Autodesk Fusion 360 part; units mm, degrees
sketch "Sketch1" plane through (0, 0, 0) normal (0, 0, 1) x (1, 0, 0)
  circle A0 centre (0, 0) radius 30
  dimension "d1" = 60
extrude "Extrude1" add sketch "Sketch1" along normal blind 5
sketch "Sketch2" plane through (0, 0, 5) normal (0, 0, 1) x (-1, 0, 0)
  circle A0 centre (0, 0) radius 30
  circle A1 centre (0, 0) radius 24.2
  dimension "d4" = 48.4
extrude "Extrude2" add sketch "Sketch2" along normal blind 25 contours A1
sketch "Sketch3" plane through (0, 0, 0) normal (0, 0, -1) x (1, 0, 0)
  circle A0 centre (0, 0) radius 30
  circle A1 centre (0, 0) radius 24.2
extrude "Extrude3" add sketch "Sketch3" along normal blind 30 contours A1
sketch "Sketch4" plane through (0, 0, 30) normal (0, 0, 1) x (-1, 0, 0)
  circle A0 centre (0, 0) radius 24.2
  circle A1 centre (0, 0) radius 22.7
  dimension "d9" = -1.5
extrude "Extrude4" cut sketch "Sketch4" against normal blind 60 contours A1
The listing builds one solid part. Answer for the finished solid, in the listing's coordinates (mm). A direction names the side the tool comes from. Coordinates: 2 decimals unless noted, no trailing zeros. Write each loop counter-clockwise with the first axis right and the second up, starting at its lowest first coordinate (ties: lowest second). Pieces come first, ordered by that corner, then holes. Notation, with made-up numbers: M 5.25,-4.5 L 12.25,-4.5 A19 ccw 12.25,25.5 Z; hole C -14.75,-18 d1. An arc over 180 degrees is marked long. Write each question's results on one line, items separated by ' | '.
Item 1: Given P1, Ø1, axis at x = -0.5, z = -17, coming from the -Y side; P2, Ø5, axis at x = -21.5, y = 22.5, coming from the -Z side; P3, Ø1, axis at y = -16, z = 0.5, coming from the -X side, each flat-ended and moving along its own axis, determine where each tip first touches the part or whether it passes through.
Answer below:
P1: y = -24.2 | P2: z = 0 | P3: x = -25.69
Item 2: Which of the six approach directions +Z, -Z, +X, -X, +Y, -Y give full straight-line access (tool end or side, diameter ignored) to faces 1 (the face through (-22.355, -9.269, 17.325)), 2 (the face through (2, 25, 0)), 3 (the face through (7, -22, -30))?
Answer below:
face 1: +Z | face 2: -Z | face 3: -Z, +X, -X, +Y, -Y
Item 3: The part is cut by section C-C on z = -25.5. Determine the outline of the cut face in (x, y).
Answer below:
outline: C 0,0 d48.4; hole C 0,0 d45.4
Item 4: The part is cut by section B-B on x = 5.5. Determine the outline of the cut face in (y, z), and give its area (3 significant figures).
Answer below:
outline: M -29.49,0 L -23.57,0 L -23.57,-30 L -22.02,-30 L -22.02,30 L -23.57,30 L -23.57,5 L -29.49,5 Z; M 22.02,-30 L 23.57,-30 L 23.57,0 L 29.49,0 L 29.49,5 L 23.57,5 L 23.57,30 L 22.02,30 Z | area: 244 mm2
Item 5: Consider probe 1 along Y at (x, z) = (0, 16); probe 2 along Z at (x, y) = (-13, -24). Determine where each line is inside the solid, lowest interval first. Write a range as [from, to].
Answer below:
probe 1: [-24.2, -22.7], [22.7, 24.2] | probe 2: [0, 5]
Item 6: The part is cut by section A-A on y = 0. Determine the outline of the cut face in (x, z), and give its area (3 significant figures).
Answer below:
outline: M -30,0 L -24.2,0 L -24.2,-30 L -22.7,-30 L -22.7,30 L -24.2,30 L -24.2,5 L -30,5 Z; M 22.7,-30 L 24.2,-30 L 24.2,0 L 30,0 L 30,5 L 24.2,5 L 24.2,30 L 22.7,30 Z | area: 238 mm2
Item 7: For a pull along Y with two mould halves and no side action, classify faces 4 (the face through (22.355, -9.269, -14.79)), 5 (the face through (-20.97, 8.69, 0.42)), 6 (the face through (2, 25, 5)) as released by +Y, released by -Y, zero draft, split by the parting line, or undercut.
Answer below:
face 4: split by the parting line | face 5: undercut | face 6: zero draft
